from build123d import *

# Parameters (mm, degrees)
SKICA1_W                = 20
SKICA1_H                = 29
P_IDAT_VYSUNUT_M1_DEPTH = 2.6
SKICA2_R                = 4
P_IDAT_VYSUNUT_M2_DEPTH = 7
SKICA3_R                = 5.5
P_IDAT_VYSUNUT_M3_DEPTH = 5.5
SKICA5_W                = 12
SKICA5_H                = 10
P_IDAT_VYSUNUT_M4_DEPTH = 25


with BuildPart() as part:
    # Skica1 → Přidat vysunutím1 (new body)
    with BuildSketch(Plane(origin=(0, 0, 0), x_dir=(1, 0, 0), z_dir=(0, 1, 0))):
        with Locations((10, 14.5)):
            Rectangle(SKICA1_W, SKICA1_H)
    extrude(amount=P_IDAT_VYSUNUT_M1_DEPTH)

    # Skica2 → Přidat vysunutím2 (add)
    with BuildSketch(Plane(origin=(0, 2.6, 0), x_dir=(1, 0, 0), z_dir=(0, 1, 0))):
        with Locations((11, 5)):
            Circle(SKICA2_R)
        with Locations((11, 22)):
            Circle(SKICA2_R)
    extrude(amount=P_IDAT_VYSUNUT_M2_DEPTH)

    # Skica3 → Přidat vysunutím3 (add)
    with BuildSketch(Plane(origin=(0, 9.6, 0), x_dir=(1, 0, 0), z_dir=(0, 1, 0))):
        with Locations((11, 22)):
            Circle(SKICA3_R)
        with Locations((11, 5)):
            Circle(SKICA3_R)
    extrude(amount=P_IDAT_VYSUNUT_M3_DEPTH)

    # Skica5 → Přidat vysunutím4 (add)
    with BuildSketch(Plane.XZ):
        with Locations((11, -22)):
            Rectangle(SKICA5_W, SKICA5_H)
        with Locations((11, -5)):
            Rectangle(SKICA5_W, SKICA5_H)
    extrude(amount=P_IDAT_VYSUNUT_M4_DEPTH)


solid = part.part
Input: part model. Units: mm. Frame: model coordinates. A direction names the side the tool comes from. Give positions to 0.01 mm unless a question says otherwise; leave off trailing zeros. Order: outer loops, then holes, each group sorted by start corner. A loop starts at its lowest first (then second) coordinate and runs counter-clockwise, first axis right, second up. Notation, with made-up numbers: (38.5, 39.5) - (53.5, 39.5) arc R19 cw to (53.5, 49.5) - close; hole circle Ø8 at (28.5, 33.25). An arc over 180 degrees is marked (long way). Answer as a JSON object with one key per item and string values. Group by question number.
Q1. Cut plane A-A, the plane y = -12. Output: boundary loops of the cut face in (x, z), then the cut area to 3 significant figures.
Q2. Cut plane B-B, the plane z = -5. Output: boundary loops of the cut face in (x, y), then the cut area to 4 significant figures.
Q3. Cut plane C-C, the plane x = 11. Output: boundary loops of the cut face in (y, z).
Q4. Mould query, pull axis Y, two halves, no side actions, for faces 1 (the face through (7.8, 6.1, -2.6)), 2 (the face through (11, 15.1, -5)), 3 (the face through (16.08, 12.31, -2.89)). Classes: pulls with the +Y half, pulls with the -Y half, needs draft (parallel to the pull), parting line crosses it, or undercut.
Q5. Set-up query: faces 4 (the face through (5, -12, -5)), 5 (the face through (11, -12, -10)), 6 (the face through (11, -12, -27)), 7 (the face through (17, -12, -22)), 8 (the face through (10.479, 6.051, -25.966)). Return all of +Z, -Z, +X, -X, +Y, -Y with unobstructed straight access to the full face (end or side cutting, diameter ignored); none if empty.
Q6. Cut plane D-D, the plane y = 11. Output: boundary loops of the cut face in (x, z).
Q7. First-contact query: pin 1 Ø11 at (y, z) = (-14.5, -7) entering from +X; pin 2 Ø1.5 at (x, y) = (12.5, -18) entering from +Z; pin 3 Ø5 at (y, z) = (-16.5, -21.5) entering from -X. Flat tips, straight axial feed; report the tip coordinate or a pass-through.
Q8. Line query: probe 1 along Z at (x, y) = (9, -15); probe 2 along Y at (x, z) = (8, -2.25); probe 3 along Y at (x, z) = (16.5, -7.5). Output: solid intervals per line, ascending.
Results:
{
 "1": {"outline": "(5, -27) - (17, -27) - (17, -17) - (5, -17) - close; (5, -10) - (17, -10) - (17, 0) - (5, 0) - close", "area": "240 mm^2"},
 "2": {"outline": "(0, 0) - (5, 0) - (5, -25) - (17, -25) - (17, 0) - (20, 0) - (20, 2.6) - (15, 2.6) - (15, 9.6) - (16.5, 9.6) - (16.5, 15.1) - (5.5, 15.1) - (5.5, 9.6) - (7, 9.6) - (7, 2.6) - (0, 2.6) - close", "area": "468.5 mm^2"},
 "3": {"outline": "(-25, -27) - (0, -27) - (0, -29) - (2.6, -29) - (2.6, -26) - (9.6, -26) - (9.6, -27.5) - (15.1, -27.5) - (15.1, -16.5) - (9.6, -16.5) - (9.6, -18) - (2.6, -18) - (2.6, -9) - (9.6, -9) - (9.6, -10.5) - (15.1, -10.5) - (15.1, 0.5) - (9.6, 0.5) - (9.6, -1) - (2.6, -1) - (2.6, 0) - (-25, 0) - (-25, -10) - (0, -10) - (0, -17) - (-25, -17) - close"},
 "4": {"face 1": "undercut", "face 2": "pulls with the +Y half", "face 3": "needs draft"},
 "5": {"face 4": "+Z, -Z, -X, -Y", "face 5": "+X, -X, -Y", "face 6": "-Z, +X, -X, -Y", "face 7": "+Z, -Z, +X, -Y", "face 8": "none"},
 "6": {"outline": "circle Ø11 at (11, -22); circle Ø11 at (11, -5)"},
 "7": {"pin 1": "x = 17", "pin 2": "z = 0", "pin 3": "x = 5"},
 "8": {"probe 1": "-27 to -17, -10 to 0", "probe 2": "-25 to 2.6, 9.6 to 15.1", "probe 3": "-25 to 2.6"}
}
